from build123d import *

# Parameters (mm, degrees)
SKETCH1_R           = 10.5
BOSS_EXTRUDE1_DEPTH = 1.85
SKETCH2_R           = 4.25
CUT_EXTRUDE1_DEPTH  = 0.5
SKETCH3_R           = 3.35
SKETCH3_R_2         = 2.9
BOSS_EXTRUDE2_DEPTH = 1.5
SKETCH4_R           = 4.5
SKETCH4_R_2         = 2.75
BOSS_EXTRUDE3_DEPTH = 3.5
SKETCH5_R           = 1.5
CUT_EXTRUDE2_DEPTH  = 5.85
SKETCH6_R           = 0.75
CUT_EXTRUDE3_DEPTH  = 6.35
CIRPATTERN1_COUNT   = 4


with BuildPart() as part:
    # Sketch1 → Boss-Extrude1 (new body)
    with BuildSketch(Plane(origin=(0, 0, 0), x_dir=(1, 0, 0), z_dir=(0, 1, 0))):
        Circle(SKETCH1_R)
    extrude(amount=BOSS_EXTRUDE1_DEPTH)

    # Sketch2 → Cut-Extrude1 (cut)
    with BuildSketch(Plane(origin=(0, 1.85, 0), x_dir=(1, 0, 0), z_dir=(0, 1, 0))):
        Circle(SKETCH2_R)
    extrude(amount=-CUT_EXTRUDE1_DEPTH, mode=Mode.SUBTRACT)

    # Sketch3 → Boss-Extrude2 (add)
    with BuildSketch(Plane(origin=(0, 1.35, 0), x_dir=(1, 0, 0), z_dir=(0, 1, 0))):
        Circle(SKETCH3_R)
        Circle(SKETCH3_R_2, mode=Mode.SUBTRACT)
    extrude(amount=BOSS_EXTRUDE2_DEPTH)

    # Sketch4 → Boss-Extrude3 (add)
    with BuildSketch(Plane.XZ):
        Circle(SKETCH4_R)
        Circle(SKETCH4_R_2, mode=Mode.SUBTRACT)
    extrude(amount=BOSS_EXTRUDE3_DEPTH)

    # Sketch5 → Cut-Extrude2 (cut, through all)
    with BuildSketch(Plane(origin=(0, 1.35, 0), x_dir=(1, 0, 0), z_dir=(0, 1, 0))):
        Circle(SKETCH5_R)
    extrude(amount=-CUT_EXTRUDE2_DEPTH, mode=Mode.SUBTRACT)

    # Sketch6 → Cut-Extrude3 (cut, through all)
    with BuildSketch(Plane(origin=(0, 1.85, 0), x_dir=(1, 0, 0), z_dir=(0, 1, 0))):
        with Locations((-3.5, 7)):
            Circle(SKETCH6_R)
        with Locations((0, 7)):
            Circle(SKETCH6_R)
        with Locations((3.5, 7)):
            Circle(SKETCH6_R)
    cut_extrude3 = extrude(amount=-CUT_EXTRUDE3_DEPTH, mode=Mode.SUBTRACT)

    # CirPattern1: Cut-Extrude3 ×4 about axis
    cirpattern1_axis = Axis((0, 0, 0), (0, 1, 0))
    for i in range(1, CIRPATTERN1_COUNT):
        add(cut_extrude3.rotate(cirpattern1_axis, i * 360 / CIRPATTERN1_COUNT), mode=Mode.SUBTRACT)


solid = part.part
For this review, take the finished solid that the model builds, in its own axes (mm). A direction names the side the tool comes from. Round coordinates to 2 decimals unless told otherwise and drop trailing zeros. Loops run counter-clockwise (first coordinate to the right, second up) from the corner with the lowest first, then second, coordinate; pieces in that order, holes last. Notation, with made-up numbers: (21, 7) - (37, 7) arc R22 ccw to (37, 29) - close; hole circle Ø5 at (-3.75, -5.5). An arc over 180 degrees is marked (long way). One line per item, written item: value. Start each with the question number.
Item 1: For faces 1 (the flat face through (1.2, 0, 1.2)), 2 (the cylindrical face through (-4.25, 0.94, -7.03)), 3 (the cylindrical face through (-2.9, 2.1, -0.1)), list the 3-axis set-ups (+Z, -Z, +X, -X, +Y, -Y) from which the entire face can be reached by the end or side of a thin tool; tool diameter is ignored.
Item 2: The part is to be moulded in two halves that separate along Z. For faces 4 (the flat face through (5, 1.85, 0)), 5 (the flat face through (1.2, 1.35, 1.2)), 6 (the cylindrical face through (-0.59, -1.73, 4.46)), say which applies: +Z half, -Z half, draft (parallel to the pull), parting line (faces both ways), or undercut.
Item 3: Take a section at B-B (z = -1). Give the boundary of the cut face in (x, y).
Item 4: Take a section at A-A (x = 6.75). Give the boundary of the cut face in (y, z), plus the area to 3 significant figures.
Item 5: Take a section at C-C (y = 1). State how many separate pieces and enclosed holes the cut face has, plus the area to 3 significant figures.
Item 6: For L1, parallel to X at y = 1.6, z = 0; L2, parallel to X at y = 0.75, z = 0, list the stretches that pass through material, from the lowest coordinate up.
Item 7: Take a section at D-D (y = -3). Give the boundary of the cut face in (x, z).
Item 8: Clearance check with flat-ended pins moving along their axes: pin 1 Ø1.5 at (x, z) = (-2, -4) entering from +Y; pin 2 Ø10.5 at (x, z) = (-4, 2.5) entering from -Y; pin 3 Ø2 at (x, z) = (-7, -3.5) entering from -Y; pin 4 Ø3 at (x, y) = (8, 1.5) entering from -Z. State where each tip first meets the part, or that it passes through.
Answer below:
1. face 1: -Y
1. face 2: +Y, -Y
1. face 3: +Y
2. face 4: draft
2. face 5: undercut
2. face 6: parting line
3. outline: (-10.45, 0) - (-4.39, 0) - (-4.39, -3.5) - (-2.56, -3.5) - (-2.56, 0) - (-1.12, 0) - (-1.12, 1.35) - (-2.72, 1.35) - (-2.72, 2.85) - (-3.2, 2.85) - (-3.2, 1.35) - (-4.13, 1.35) - (-4.13, 1.85) - (-10.45, 1.85) - close; (1.12, 0) - (2.56, 0) - (2.56, -3.5) - (4.39, -3.5) - (4.39, 0) - (10.45, 0) - (10.45, 1.85) - (4.13, 1.85) - (4.13, 1.35) - (3.2, 1.35) - (3.2, 2.85) - (2.72, 2.85) - (2.72, 1.35) - (1.12, 1.35) - close
4. outline: (0, -8.04) - (1.85, -8.04) - (1.85, -4.21) - (0, -4.21) - close; (0, -2.79) - (1.85, -2.79) - (1.85, -0.71) - (0, -0.71) - close; (0, 0.71) - (1.85, 0.71) - (1.85, 2.79) - (0, 2.79) - close; (0, 4.21) - (1.85, 4.21) - (1.85, 8.04) - (0, 8.04) - close
4. area: 21.9 mm2
5. separate pieces: 1
5. enclosed holes: 13
5. area: 318 mm2
6. L1: x = -10.5 to -7.75, -6.25 to -4.25, -3.35 to -2.9, 2.9 to 3.35, 4.25 to 6.25, 7.75 to 10.5
6. L2: x = -10.5 to -7.75, -6.25 to -1.5, 1.5 to 6.25, 7.75 to 10.5
7. outline: circle Ø9 at (0, 0); hole circle Ø5.5 at (0, 0)
8. pin 1: stops at y = 1.85
8. pin 2: stops at y = -3.5
8. pin 3: stops at y = 0
8. pin 4: stops at z = -8.25
